Geometry: see drawing. Coordinates: mm, zero at the bounding-box minimum. A direction names the side the tool comes from. Coordinates: 2 decimals unless noted, no trailing zeros. Write each loop counter-clockwise with the first axis right and the second up, starting at its lowest first coordinate (ties: lowest second). Pieces come first, ordered by that corner, then holes. Notation, with made-up numbers: (-30, 38.25) - (23, 38.25) arc R12 ccw to (23, 53.25) - close; hole circle Ø8 at (1.25, 12.25). An arc over 180 degrees is marked (long way). Use a Markdown table: item, result. Add a question column.
Q1. Section query B-B (z = 69). Return the cut outline in (x, y) (1 decimal), then the cut area to 3 significant figures.
Q2. Mould query, pull axis X, two halves, no side actions, for the marked faces 1, 2, 3 and 4. Classes: released by +X, released by -X, zero draft, split by the parting line, or undercut.
Q3. Section query D-D (y = 96). Return the cut outline in (x, z) (1 decimal), then the cut area to 3 significant figures.
Q4. Material intervals for probe 1 along Y at (x, z) = (52.5, 51); probe 2 along Y at (x, z) = (59.5, 72.5); probe 3 along X at (y, z) = (96.5, 45.5) (1 decimal), sorted ascending. Write a range as from..to.
Q5. Set-up query: the marked faces 5, 6, 7 and 8. Return all of +Z, -Z, +X, -X, +Y, -Y with unobstructed straight access to the full face (end or side cutting, diameter ignored); none if empty.
Q6. Section query C-C (x = 105). Return the cut outline in (y, z) (1 decimal).
Q7. Pin query (flat end, axial travel): P1, Ø1, axis at x = 67.5, y = 66.5, coming from the -Z side; P2, Ø6.5, axis at y = 118, z = 77.5, coming from the -X side (1 decimal); P3, Ø8, axis at x = 111, y = 23, coming from the +Z side; P4, Ø23.5, axis at x = 63.5, y = 72, coming from the +Z side. Return the tip coordinate at first contact, or that it passes through.
Q8. Section query A-A (z = 99). Return the cut outline in (x, y) (1 decimal).
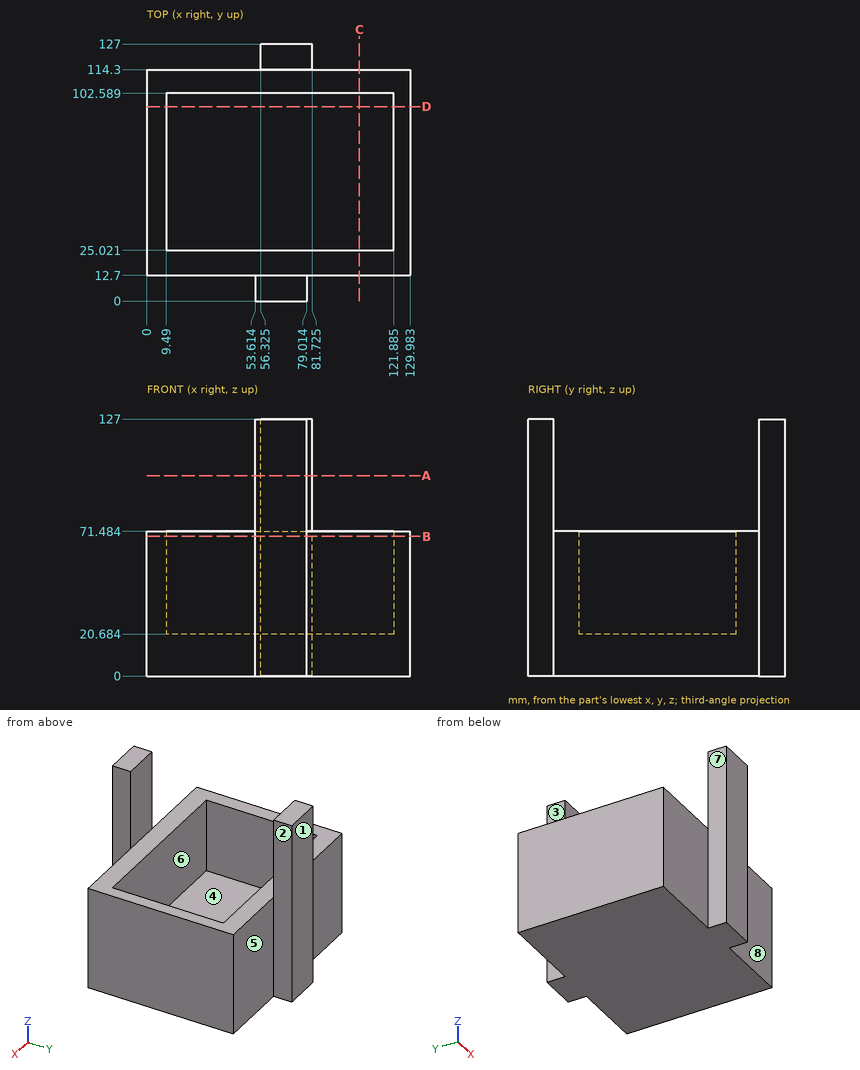
Values follow:
| question | item | result |
|---|---|---|
| 1 | outline | (0, 12.7) - (53.6, 12.7) - (53.6, 0) - (79, 0) - (79, 12.7) - (130, 12.7) - (130, 114.3) - (81.7, 114.3) - (81.7, 127) - (56.3, 127) - (56.3, 114.3) - (0, 114.3) - close; hole (9.5, 25) - (121.9, 25) - (121.9, 102.6) - (9.5, 102.6) - close |
| 1 | area | 5,130 mm2 |
| 2 | face 1 | zero draft |
| 2 | face 2 | released by +X |
| 2 | face 3 | released by -X |
| 2 | face 4 | undercut |
| 3 | outline | (0, 0) - (130, 0) - (130, 71.5) - (121.9, 71.5) - (121.9, 20.7) - (9.5, 20.7) - (9.5, 71.5) - (0, 71.5) - close |
| 3 | area | 3,580 mm2 |
| 4 | probe 1 | 12.7..25.02, 102.59..114.3 |
| 4 | probe 2 | 0..12.7, 114.3..127 |
| 4 | probe 3 | 0..9.5, 121.9..130 |
| 5 | face 5 | +Z, -Z, +X, +Y |
| 5 | face 6 | +Z |
| 5 | face 7 | +Z, -Z, -X, -Y |
| 5 | face 8 | +Z, -Z, +X, -Y |
| 6 | outline | (12.7, 0) - (114.3, 0) - (114.3, 71.5) - (102.6, 71.5) - (102.6, 20.7) - (25, 20.7) - (25, 71.5) - (12.7, 71.5) - close |
| 7 | P1 | z = 0 |
| 7 | P2 | x = 56.3 |
| 7 | P3 | z = 71.48 |
| 7 | P4 | z = 20.68 |
| 8 | outline | (53.6, 0) - (79, 0) - (79, 12.7) - (53.6, 12.7) - close; (56.3, 114.3) - (81.7, 114.3) - (81.7, 127) - (56.3, 127) - close |
